Answer from the drawing. Dimensions are ordinates in mm from the lowest x, y and z of the part. A direction names the side the tool comes from. Give positions to 0.01 mm unless a question says otherwise; leave off trailing zeros. Loops run counter-clockwise (first coordinate to the right, second up) from the corner with the lowest first, then second, coordinate; pieces in that order, holes last. Notation, with made-up numbers: M 87.25,-8.5 L 140.25,-8.5 A28 ccw 140.25,26.5 Z; hole C 12,-38.75 d10. An arc over 180 degrees is marked long. Return JSON: item names as keys, results as strings. Group by question number.
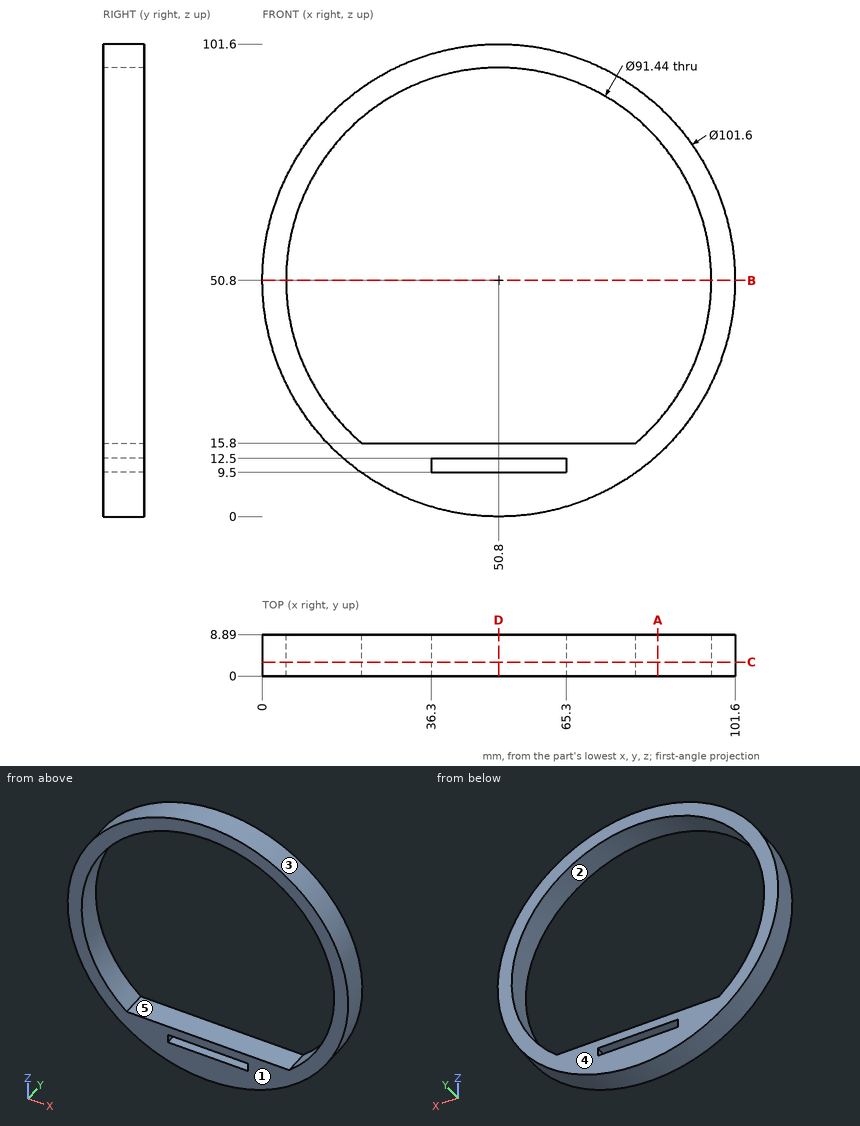
1. The mould has two halves that part along Z. Classify the marked faces 1, 2 and 3: +Z half, -Z half, draft (parallel to the pull), parting line (faces both ways), or undercut.
2. Find section D-D (x = 50.8). Write down the section's boundary in (y, z).
3. Find section A-A (x = 85). Write down the section's boundary in (y, z), and give its area (3 significant figures).
4. For the marked faces 4 and 5, determine the directions among +Z, -Z, +X, -X, +Y, -Y from which every point of the face is accessible in a straight line to the end or side of a thin tool.
5. Straight lines are drawn through the part: line 1 along X through (y, z) = (3.5, 50.8); line 2 along Z through (x, y) = (64.5, 0.5); line 3 along X through (y, z) = (4.75, 80). For each, find the intervals that lie inside material, in ascending order.
6. Flat-ended cylindrical pins translate along their axes: P1, Ø0.9, axis at y = 2.5, z = 11, coming from the -X side; P2, Ø1, axis at x = 37, y = 4.5, coming from the -Z side; P3, Ø4.5, axis at x = 54.5, y = 6.5, coming from the -Z side. Find the tip coordinate at first contact, or state that the pin passes through.
7. Find section C-C (y = 3). Write down the section's boundary in (x, z), and give its area (3 significant figures).
8. Find section B-B (z = 50.8). Write down the section's boundary in (x, y), and give its area (3 significant figures).
Result:
{
 "1": {"face 1": "draft", "face 2": "undercut", "face 3": "parting line"},
 "2": {"outline": "M 0,0 L 8.89,0 L 8.89,9.5 L 0,9.5 Z; M 0,12.5 L 8.89,12.5 L 8.89,15.8 L 0,15.8 Z; M 0,96.52 L 8.89,96.52 L 8.89,101.6 L 0,101.6 Z"},
 "3": {"outline": "M 0,13.24 L 8.89,13.24 L 8.89,20.46 L 0,20.46 Z; M 0,81.14 L 8.89,81.14 L 8.89,88.36 L 0,88.36 Z", "area": "128 mm2"},
 "4": {"face 4": "+Z, -Z, +X, -X, +Y", "face 5": "+Y, -Y"},
 "5": {"line 1": "x = 0 to 5.08, 96.52 to 101.6", "line 2": "z = 1.88 to 9.5, 12.5 to 15.8, 94.42 to 99.72", "line 3": "x = 9.23 to 15.62, 85.98 to 92.37"},
 "6": {"P1": "stops at x = 18.67", "P2": "stops at z = 1.77", "P3": "stops at z = 0.02"},
 "7": {"outline": "C 50.8,50.8 d101.6; hole M 21.38,15.8 L 80.22,15.8 A45.72 ccw long Z; hole M 36.3,9.5 L 65.3,9.5 L 65.3,12.5 L 36.3,12.5 Z", "area": "1,880 mm2"},
 "8": {"outline": "M 0,0 L 5.08,0 L 5.08,8.89 L 0,8.89 Z; M 96.52,0 L 101.6,0 L 101.6,8.89 L 96.52,8.89 Z", "area": "90.3 mm2"}
}
